The listing builds one solid part. Answer for the finished solid, in the listing's coordinates (mm). A direction names the side the tool comes from. Round coordinates to 2 decimals unless told otherwise and drop trailing zeros. One line per item, written item: value. Start each with the question number.
(1) For faces 1 (the flat face through (-77, 3, 257.175)), 2 (the flat face through (-1, 3, 254)), 3 (the flat face through (133, 3, 254)), 4 (the flat face through (152.4, 3, 216)), 5 (the flat face through (-134, 3, 254)), determine the directions among +Z, -Z, +X, -X, +Y, -Y from which every point of the face is accessible in a straight line to the end or side of a thin tool.
(2) Consider probe 1 along Z at (x, y) = (0, 5) (1 decimal); probe 2 along X at (y, z) = (1.5, 0); probe 3 along X at (y, z) = (5.5, 11.5). Determine where each line is inside the solid, lowest interval first.
(3) Given P1, Ø1.9, axis at x = -11.5, y = 3, coming from the +Z side, flat-ended and moving along its own axis, determine where the tip first touches the part or whether it passes through.
(4) For a pull along X with two mould halves and no side action, classify faces 6 (the flat face through (-152.4, 3, 215)), 7 (the cylindrical face through (14.274, 3.131, -0.628)), 8 (the flat face through (2, 6.35, 146)) as released by +X, released by -X, zero draft, split by the parting line, or undercut.
Autodesk Inventor part; units mm, degrees
ref_plane "YZ Plane" through (0, 0, 0) normal (1, 0, 0) x (0, 1, 0)
ref_plane "XZ Plane" through (0, 0, 0) normal (0, 1, 0) x (-1, 0, 0)
ref_plane "XY Plane" through (0, 0, 0) normal (0, 0, 1) x (1, 0, 0)
sketch "Sketch1" plane through (0, 0, 0) normal (0, 1, 0) x (-1, 0, 0)
  line L0 (0, -234.315) -> (0, 339.09)
  line L1 (-213.36, 0) -> (213.36, 0)
  line L2 (213.36, 0) -> (-213.36, 0)
  line L3 (0, -234.315) -> (0, 339.09)
  line L4 (152.4, 254) -> (-152.4, 254)
  line L5 (-152.4, 254) -> (-152.4, 0)
  line L6 (152.4, 0) -> (152.4, 254)
  arc A0 (-152.4, 0) -> (152.4, 0) centre (0, 0) ccw
  line L7 (111.125, 254) -> (41.275, 254) construction
  line L8 (111.125, 257.175) -> (41.275, 257.175)
  line L9 (41.275, 250.825) -> (111.125, 250.825)
  arc A1 (111.125, 250.825) -> (111.125, 257.175) centre (111.125, 254) ccw
  arc A2 (41.275, 257.175) -> (41.275, 250.825) centre (41.275, 254) ccw
  line L10 (-41.275, 254) -> (-111.125, 254) construction
  line L11 (-41.275, 257.175) -> (-111.125, 257.175)
  line L12 (-111.125, 250.825) -> (-41.275, 250.825)
  arc A3 (-41.275, 250.825) -> (-41.275, 257.175) centre (-41.275, 254) ccw
  arc A4 (-111.125, 257.175) -> (-111.125, 250.825) centre (-111.125, 254) ccw
  circle A5 centre (0, 0) radius 14.2875
  point P0 (76.2, 254)
  point P1 (-76.2, 254)
  point P2 (0, -152.4)
  point P3 (114.3, 254)
  point P4 (38.1, 254)
  dimension "d2" = 69.85
  dimension "d3" = 6.35
  dimension "d4" = 69.85
  dimension "d5" = 6.35
  dimension "d7" = 76.2
  dimension "d8" = 304.8
  dimension "d9" = 76.2
  dimension "d10" = 28.575
  dimension "d11" = 406.4
  dimension "d15" = 76.2
extrude "Extrusion1" add sketch "Sketch1" along normal blind 6.35 contours A0 L1 A5 L0 | L0 A5 L1 A0 | L5 L4 A4 L12 A3 L0 A5 L1 | L1 A5 L0 L4 A2 L9 A1 L6 | A4 L11 A3 L4 | L4 A3 L12 A4 | A1 L9 A2 L4 | L4 A2 L8 A1
sketch "Sketch5" plane through (0, 6.35, 0) normal (0, 1, 0) x (1, 0, 0)
  circle A0 centre (0, 0) radius 14.2875
  line L0 (-38.1, -254) -> (38.1, -254)
  arc A1 (38.1, -254) -> (41.275, -257.175) centre (41.275, -254) ccw
  line L1 (41.275, -257.175) -> (111.125, -257.175)
  arc A2 (111.125, -257.175) -> (114.3, -254) centre (111.125, -254) ccw
  line L2 (114.3, -254) -> (152.4, -254)
  line L3 (152.4, -254) -> (152.4, 0)
  arc A3 (152.4, 0) -> (-152.4, 0) centre (0, 0) ccw
  line L4 (-152.4, 0) -> (-152.4, -254)
  line L5 (-152.4, -254) -> (-114.3, -254)
  arc A4 (-114.3, -254) -> (-111.125, -257.175) centre (-111.125, -254) ccw
  line L6 (-111.125, -257.175) -> (-41.275, -257.175)
  arc A5 (-41.275, -257.175) -> (-38.1, -254) centre (-41.275, -254) ccw
  line L7 (-152.4, -254) -> (152.4, -254)
  line L8 (152.4, -254) -> (152.4, -177.8)
  line L9 (152.4, -177.8) -> (-152.4, -177.8)
  line L10 (-152.4, -177.8) -> (-152.4, -254)
  line L11 (-152.4, -177.8) -> (152.4, -177.8)
  line L12 (152.4, -177.8) -> (152.4, 0)
  line L13 (-152.4, 0) -> (-152.4, -177.8)
  arc A6 (152.4, 0) -> (-152.4, 0) centre (0, 0) ccw
  line L14 (-152.4, 0) -> (-152.4, -254)
  line L15 (-152.4, -177.8) -> (-152.4, 0) construction
  line L16 (-152.4, 0) -> (0, 152.4) construction
  line L17 (0, 152.4) -> (152.4, 0) construction
  line L18 (152.4, 0) -> (152.4, -177.8) construction
  line L19 (152.4, -254) -> (152.4, 0)
  spline S0 degree 4 poles (-152.4, -177.8) (-152.4, 0) (0, 152.4) (152.4, 0) (152.4, -177.8) knots 1 1 1 1 1 2 2 2 2 2
  dimension "d20" = 304.8
  dimension "d21" = 76.2
extrude "Extrusion2" cut sketch "Sketch5" against normal blind 25.4 contours L4 A3 L3 S0
properties part number "turretSidePlateTwo"
Recorded:
1. face 1: +Z, +X, -X, +Y, -Y
1. face 2: +Z, +Y, -Y
1. face 3: +Z, +X, +Y, -Y
1. face 4: +Z, -Z, +X, +Y, -Y
1. face 5: +Z, -X, +Y, -Y
2. probe 1: z = -34.9 to -14.3, 14.3 to 254
2. probe 2: x = -82.57 to -14.29, 14.29 to 82.57
2. probe 3: x = -93.9 to -8.48, 8.48 to 93.9
3. P1: stops at z = 254
4. face 6: released by -X
4. face 7: undercut
4. face 8: zero draft
